Answer from the drawing. Dimensions are ordinates in mm from the lowest x, y and z of the part. A direction names the side the tool comes from. Coordinates: 2 decimals unless noted, no trailing zeros. Write each loop counter-clockwise with the first axis right and the second up, starting at its lowest first coordinate (ties: lowest second). Pieces come first, ordered by that corner, then holes. Notation, with made-up numbers: (38.25, 29) -> (95.25, 29) arc R30 ccw to (95.25, 66) -> close; hole circle Ø10 at (79, 38.5). An arc over 180 degrees is marked (long way). Return JSON: item names as keys, results as strings.
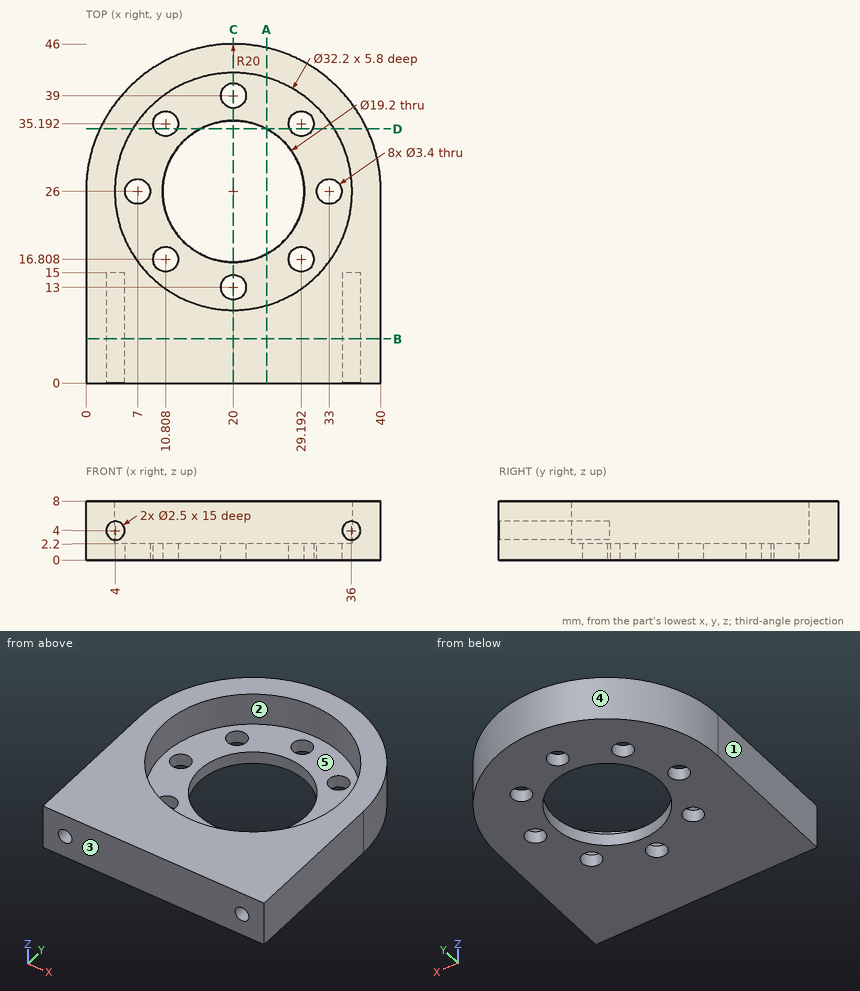
1. Consider L1, parallel to Y at x = 20.5, z = 4.75; L2, parallel to Y at x = 28.5, z = 0.5 (1 decimal); L3, parallel to Y at x = 9, z = 2.25 (1 decimal). Determine where each line is inside the solid, lowest interval first.
Taken from the geometry:
{"L1": "y = 0 to 9.91, 42.09 to 45.99", "L2": "y = 0 to 15.3, 18.4 to 21.5, 30.5 to 33.6, 36.7 to 44.1", "L3": "y = 0 to 14.2, 37.8 to 42.7"}
2. The part is cut by section C-C (x = 20). Determine the outline of the cut face in (y, z), then the cut area to 3 significant figures.
Taken from the geometry:
{"outline": "(0, 0) -> (11.3, 0) -> (11.3, 2.2) -> (9.9, 2.2) -> (9.9, 8) -> (0, 8) -> close; (14.7, 0) -> (16.4, 0) -> (16.4, 2.2) -> (14.7, 2.2) -> close; (35.6, 0) -> (37.3, 0) -> (37.3, 2.2) -> (35.6, 2.2) -> close; (40.7, 0) -> (46, 0) -> (46, 8) -> (42.1, 8) -> (42.1, 2.2) -> (40.7, 2.2) -> close", "area": "124 mm2"}
3. The part is cut by section A-A (x = 24.5). Determine the outline of the cut face in (y, z), then the cut area to 3 significant figures.
Taken from the geometry:
{"outline": "(0, 0) -> (17.52, 0) -> (17.52, 2.2) -> (10.54, 2.2) -> (10.54, 8) -> (0, 8) -> close; (34.48, 0) -> (45.49, 0) -> (45.49, 8) -> (41.46, 8) -> (41.46, 2.2) -> (34.48, 2.2) -> close", "area": "147 mm2"}
4. Flat-ended cylindrical pins translate along their axes: pin 1 Ø2 at (x, y) = (20, 13) entering from -Z; pin 2 Ø1.5 at (x, z) = (16.5, 4) entering from +Y; pin 3 Ø12 at (x, y) = (16, 33) entering from +Z; pin 4 Ø2 at (x, z) = (4, 4) entering from +Y. Find the tip coordinate at first contact, or state that the pin passes through.
Taken from the geometry:
{"pin 1": "passes through", "pin 2": "stops at y = 45.81", "pin 3": "stops at z = 2.2", "pin 4": "stops at y = 39.23"}
5. A tool of negligible diameter and unlimited length cuts with its end or side. For the marked faces 4 and 5, from which of +Z, -Z, +X, -X, +Y, -Y can it reach the whole face along a straight path? Write none if from no direction.
Taken from the geometry:
{"face 4": "+Z, -Z, +Y", "face 5": "+Z"}
6. The part is cut by section B-B (y = 6). Determine the outline of the cut face in (x, z), then the cut area to 3 significant figures.
Taken from the geometry:
{"outline": "(0, 0) -> (40, 0) -> (40, 8) -> (0, 8) -> close; hole circle Ø2.5 at (4, 4); hole circle Ø2.5 at (36, 4)", "area": "310 mm2"}
7. For a pull along Y with two mould halves and no side action, classify the marked faces 1, 2 and 3 as +Y half, -Y half, draft (parallel to the pull), parting line (faces both ways), or undercut.
Taken from the geometry:
{"face 1": "draft", "face 2": "undercut", "face 3": "-Y half"}
8. The part is cut by section D-D (y = 34.5). Determine the outline of the cut face in (x, z) (1 decimal).
Taken from the geometry:
{"outline": "(1.9, 0) -> (9.3, 0) -> (9.3, 2.2) -> (6.3, 2.2) -> (6.3, 8) -> (1.9, 8) -> close; (12.4, 0) -> (15.5, 0) -> (15.5, 2.2) -> (12.4, 2.2) -> close; (24.5, 0) -> (27.6, 0) -> (27.6, 2.2) -> (24.5, 2.2) -> close; (30.7, 0) -> (38.1, 0) -> (38.1, 8) -> (33.7, 8) -> (33.7, 2.2) -> (30.7, 2.2) -> close"}
